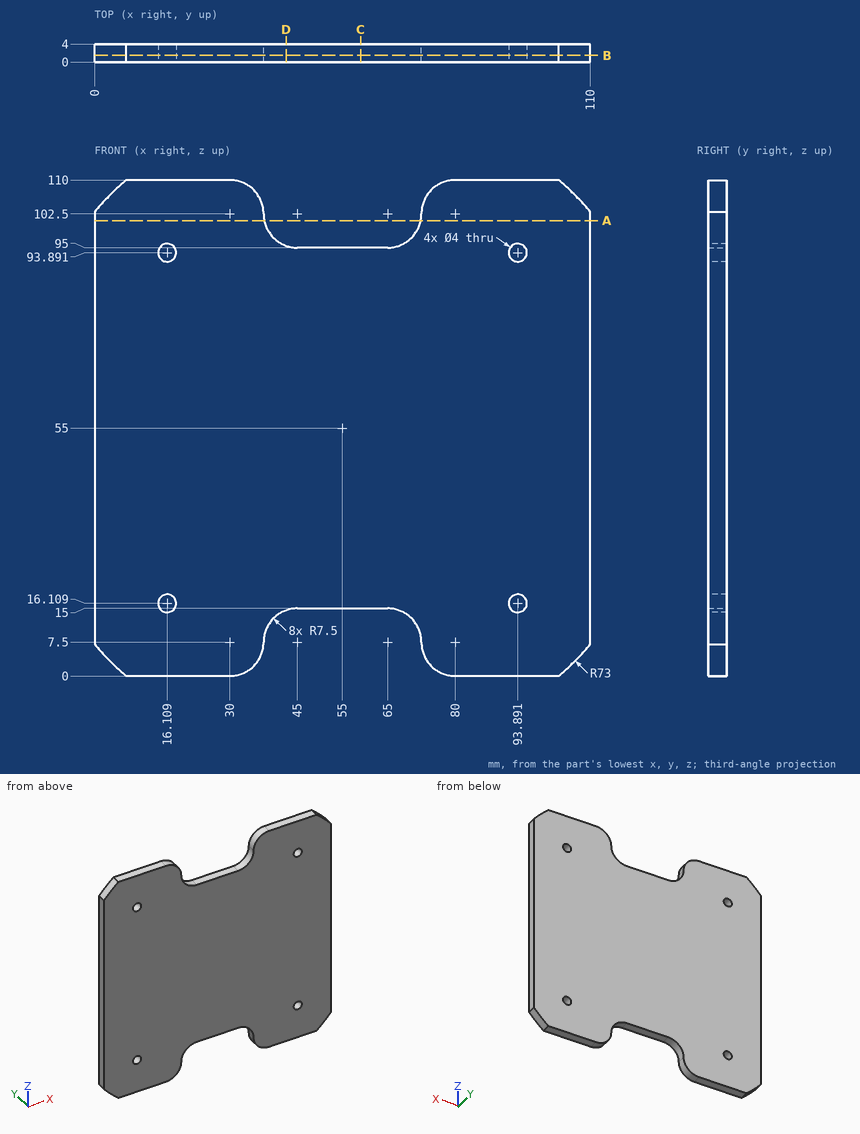
Input: dimensioned drawing with shaded views. Units: mm. Origin: part minimum x, y, z. Round coordinates to 2 decimals unless told otherwise and drop trailing zeros. Order: outer loops, then holes, each group sorted by start corner. A loop starts at its lowest first (then second) coordinate and runs counter-clockwise, first axis right, second up. Notation, with made-up numbers: (68, -24) - (107, -24) arc R26 cw to (107, 6) - close; hole circle Ø8 at (22.5, 23.5). An arc over 180 degrees is marked (long way). Answer as a JSON object with one key per item and string values. Group by question number.
(1) Pin query (flat end, axial travel): P1, Ø2, axis at x = 51, y = 1.5, coming from the -Z side. Return the tip coordinate at first contact, or that it passes through.
(2) Cut plane D-D (x = 42.5). Return loops of the section in (y, z), then the cut area to 3 significant figures.
(3) Material intervals for probe 1 along X at (y, z) = (3, 104.5); probe 2 along Z at (x, y) = (60.5, 1.5); probe 3 along Z at (x, y) = (76, 1.6), sorted ascending. Write a range as from..to.
(4) Cut plane A-A (z = 101). Return loops of the section in (x, y).
(5) Cut plane C-C (x = 59). Return loops of the section in (y, z), then the cut area to 3 significant figures.
(6) Cut plane B-B (y = 1.5). Return loops of the section in (x, z), then the cut area to 3 significant figures.
Here are the results:
{
 "1": {"P1": "stops at z = 15"},
 "2": {"outline": "(0, 14.57) - (4, 14.57) - (4, 95.43) - (0, 95.43) - close", "area": "323 mm^2"},
 "3": {"probe 1": "x = 1.35..37.23, 72.77..108.65", "probe 2": "z = 15..95", "probe 3": "z = 1.16..108.84"},
 "4": {"outline": "(0, 0) - (37.65, 0) - (37.65, 4) - (0, 4) - close; (72.35, 0) - (110, 0) - (110, 4) - (72.35, 4) - close"},
 "5": {"outline": "(0, 15) - (4, 15) - (4, 95) - (0, 95) - close", "area": "320 mm^2"},
 "6": {"outline": "(0, 7) arc R73 ccw to (7, 0) - (30, 0) arc R7.5 ccw to (37.5, 7.5) arc R7.5 cw to (45, 15) - (65, 15) arc R7.5 cw to (72.5, 7.5) arc R7.5 ccw to (80, 0) - (103, 0) arc R73 ccw to (110, 7) - (110, 103) arc R73 ccw to (103, 110) - (80, 110) arc R7.5 ccw to (72.5, 102.5) arc R7.5 cw to (65, 95) - (45, 95) arc R7.5 cw to (37.5, 102.5) arc R7.5 ccw to (30, 110) - (7, 110) arc R73 ccw to (0, 103) - close; hole circle Ø4 at (16.11, 16.11); hole circle Ø4 at (16.11, 93.89); hole circle Ø4 at (93.89, 16.11); hole circle Ø4 at (93.89, 93.89)", "area": "10,900 mm^2"}
}
